Source: CAD feature listing. Evaluate the final solid. Frame: model axes, mm. A direction names the side the tool comes from. Coordinates: 2 decimals unless noted, no trailing zeros. Write each loop counter-clockwise with the first axis right and the second up, starting at its lowest first coordinate (ties: lowest second). Pieces come first, ordered by that corner, then holes. Notation, with made-up numbers: (13.25, 8) -> (42.25, 8) arc R29 cw to (42.25, 44) -> close; hole circle Ø8 at (78.5, 69). An arc over 180 degrees is marked (long way). Write item = value, one per line.
from build123d import *

# Parameters (mm, degrees)
SKETCH1_W                = 177
SKETCH1_H                = 62
BOSS_EXTRUDE1_DEPTH      = 70
FILLET1_R                = 25
SKETCH3_W                = 19
SKETCH3_H                = 17
CUT_EXTRUDE1_DEPTH       = 70
CUT_EXTRUDE5_DEPTH       = 64
BOSS_EXTRUDE7_DEPTH      = 33
SKETCH16_W               = 5
SKETCH16_H               = 5
BOSS_EXTRUDE8_DEPTH      = 40
SKETCH11_R               = 25
CUT_EXTRUDE9_DEPTH       = 5.5
SKETCH22_R               = 28.5
BOSS_EXTRUDE20_DEPTH     = 21
BOSS_EXTRUDE21_DEPTH     = 10
BOSS_EXTRUDE22_DEPTH     = 40
SKETCH26_R               = 25
SKETCH26_W               = 19
SKETCH26_H               = 17
BOSS_EXTRUDE23_DEPTH     = 1
SKETCH27_W               = 40
SKETCH27_H               = 10
CUT_EXTRUDE12_DEPTH      = 10
SKETCH28_W               = 10
SKETCH28_H               = 10
CUT_EXTRUDE13_DEPTH      = 5
SKETCH30_W               = 194.337314874
SKETCH30_H               = 68.122542634
CUT_EXTRUDE14_DEPTH      = 0.1
CUT_EXTRUDE17_DEPTH      = 58
CUT_EXTRUDE17_DEPTH_BACK = 45
SKETCH26_3_R             = 25
SKETCH26_3_W             = 19
SKETCH26_3_H             = 17
CUT_EXTRUDE25_START      = -21.9
CUT_EXTRUDE25_DEPTH      = 21.9
SKETCH38_W               = 8
SKETCH38_H               = 8
BOSS_EXTRUDE26_DEPTH     = 12
SKETCH41_R               = 3.6
CUT_EXTRUDE28_DEPTH      = 5
SKETCH44_R               = 2.1
CUT_EXTRUDE29_DEPTH      = 8
CUT_EXTRUDE30_START      = -3
SKETCH22_2_R             = 28.5
CUT_EXTRUDE30_DEPTH      = 40
SKETCH45_W               = 19.955287375
SKETCH45_H               = 24.166036088
CUT_EXTRUDE31_DEPTH      = 112


with BuildPart() as part:
    # Sketch1 → Boss-Extrude1 (new body)
    with BuildSketch(Plane(origin=(0, 0, 0), x_dir=(1, 0, 0), z_dir=(0, 1, 0))):
        with Locations((88.5, 31)):
            Rectangle(SKETCH1_W, SKETCH1_H)
    extrude(amount=BOSS_EXTRUDE1_DEPTH)

    # Fillet1
    fillet1_edges = [part.edges().sort_by_distance(p)[0] for p in [
        (0, 35, -62),
        (177, 35, -62),
        (177, 35, 0),
        (0, 35, 0),
    ]]
    fillet(fillet1_edges, radius=FILLET1_R)

    # Sketch3 → Cut-Extrude1 (cut)
    with BuildSketch(Plane(origin=(0, 70, 0), x_dir=(1, 0, 0), z_dir=(0, 1, 0))):
        with Locations((147.5, 39.5)):
            Rectangle(SKETCH3_W, SKETCH3_H)
    extrude(amount=-CUT_EXTRUDE1_DEPTH, mode=Mode.SUBTRACT)

    # Sketch9 → Cut-Extrude5 (cut)
    with BuildSketch(Plane(origin=(0, 67, 0), x_dir=(1, 0, 0), z_dir=(0, 1, 0))):
        with BuildLine():
            Line((25, 59), (152, 59))
            ThreePointArc((152, 59), (167.556349186, 52.556349186), (174, 37))
            Line((174, 37), (174, 25))
            ThreePointArc((174, 25), (167.556349186, 9.443650814), (152, 3))
            Line((152, 3), (25, 3))
            ThreePointArc((25, 3), (9.443650814, 9.443650814), (3, 25))
            Line((3, 25), (3, 37))
            ThreePointArc((3, 37), (9.443650814, 52.556349186), (25, 59))
        make_face()
    extrude(amount=-CUT_EXTRUDE5_DEPTH, mode=Mode.SUBTRACT)

    # Sketch15 → Boss-Extrude7 (add)
    with BuildSketch(Plane.XZ):
        Polygon((125, -7), (121, -3), (119, -3), (119, -7.5), (125, -7.5), align=None)
        Polygon((137, -7), (137, -7.5), (143, -7.5), (143, -3), (141, -3), align=None)
    extrude(amount=-BOSS_EXTRUDE7_DEPTH)

    # Sketch16 → Boss-Extrude8 (add)
    with BuildSketch(Plane.XZ):
        with Locations((58.5, -5.5)):
            Rectangle(SKETCH16_W, SKETCH16_H)
        Polygon((61, -40.5), (61, -44), (101, -44), (101, -40.5), (106, -40.5), (106, -59), (56, -59), (56, -40.5), align=None)
        with Locations((104.5, -5.5)):
            Rectangle(SKETCH16_W, SKETCH16_H)
    extrude(amount=-BOSS_EXTRUDE8_DEPTH)

    # Sketch11 → Cut-Extrude9 (cut)
    with BuildSketch(Plane.XZ):
        with Locations(Location((31, -31, 0), (0, 0, 270))):
            Circle(SKETCH11_R)
    extrude(amount=-CUT_EXTRUDE9_DEPTH, mode=Mode.SUBTRACT)

    # Sketch22 → Boss-Extrude20 (add)
    with BuildSketch(Plane(origin=(0, 70, 0), x_dir=(1, 0, 0), z_dir=(0, 1, 0))):
        with Locations((31, 31)):
            Circle(SKETCH22_R)
    extrude(amount=-BOSS_EXTRUDE20_DEPTH)

    # Sketch24 → Boss-Extrude21 (add)
    with BuildSketch(Plane.XZ):
        Polygon((123.5, -7.5), (125, -7.5), (125, -29.5), (137, -29.5), (137, -7.5), (138.5, -7.5), (138.5, -35.5), (123.5, -35.5), align=None)
    extrude(amount=-BOSS_EXTRUDE21_DEPTH)

    # Sketch25 → Boss-Extrude22 (add)
    with BuildSketch(Plane.XZ):
        Polygon((134.5, -35.5), (134.5, -31.5), (124.5, -31.5), (124.5, -45.5), (128.5, -45.5), (128.5, -35.5), align=None)
        Polygon((160.5, -35.5), (166.5, -35.5), (166.5, -45.5), (170.5, -45.5), (170.5, -31.5), (160.5, -31.5), align=None)
    extrude(amount=-BOSS_EXTRUDE22_DEPTH)

    # Sketch26 → Boss-Extrude23 (add)
    with BuildSketch(Plane.XZ):
        with BuildLine():
            Line((25, 0), (152, 0))
            ThreePointArc((152, 0), (169.67766953, -7.32233047), (177, -25))
            Line((177, -25), (177, -37))
            ThreePointArc((177, -37), (169.67766953, -54.67766953), (152, -62))
            Line((152, -62), (25, -62))
            ThreePointArc((25, -62), (7.32233047, -54.67766953), (0, -37))
            Line((0, -37), (0, -25))
            ThreePointArc((0, -25), (7.32233047, -7.32233047), (25, 0))
        make_face()
        with Locations(Location((31, -31, 0), (0, 0, 270))):
            Circle(SKETCH26_R, mode=Mode.SUBTRACT)
        with Locations((147.5, -39.5)):
            Rectangle(SKETCH26_W, SKETCH26_H, mode=Mode.SUBTRACT)
    extrude(amount=BOSS_EXTRUDE23_DEPTH)

    # Sketch27 → Cut-Extrude12 (cut)
    with BuildSketch(Plane.ZY):
        with Locations((-31, 34.5)):
            Rectangle(SKETCH27_W, SKETCH27_H)
    extrude(amount=-CUT_EXTRUDE12_DEPTH, mode=Mode.SUBTRACT)

    # Sketch28 → Cut-Extrude13 (cut)
    with BuildSketch(Plane.XZ.offset(1)):
        with Locations((115, -54)):
            Rectangle(SKETCH28_W, SKETCH28_H)
    extrude(amount=-CUT_EXTRUDE13_DEPTH, mode=Mode.SUBTRACT)

    # Sketch30 → Cut-Extrude14 (cut)
    with BuildSketch(Plane(origin=(0, 67, 0), x_dir=(1, 0, 0), z_dir=(0, 1, 0))):
        with Locations((88.376869027, 31.076383763)):
            Rectangle(SKETCH30_W, SKETCH30_H)
        with BuildLine():
            Line((25, 58), (152, 58))
            ThreePointArc((152, 58), (166.849242405, 51.849242405), (173, 37))
            Line((173, 37), (173, 25))
            ThreePointArc((173, 25), (166.849242405, 10.150757595), (152, 4))
            Line((152, 4), (25, 4))
            ThreePointArc((25, 4), (10.150757595, 10.150757595), (4, 25))
            Line((4, 25), (4, 37))
            ThreePointArc((4, 37), (10.150757595, 51.849242405), (25, 58))
        make_face(mode=Mode.SUBTRACT)
    extrude(amount=-CUT_EXTRUDE14_DEPTH, mode=Mode.SUBTRACT)

    # Sketch26<3> → Cut-Extrude17 (cut, two sides: drawn at the far end of the back side and taken through both)
    with BuildSketch(Plane.XZ.offset(-CUT_EXTRUDE17_DEPTH_BACK)):
        with BuildLine():
            Line((25, 0), (152, 0))
            ThreePointArc((152, 0), (169.67766953, -7.32233047), (177, -25))
            Line((177, -25), (177, -37))
            ThreePointArc((177, -37), (169.67766953, -54.67766953), (152, -62))
            Line((152, -62), (25, -62))
            ThreePointArc((25, -62), (7.32233047, -54.67766953), (0, -37))
            Line((0, -37), (0, -25))
            ThreePointArc((0, -25), (7.32233047, -7.32233047), (25, 0))
        make_face()
        with Locations((31, -31)):
            Circle(SKETCH26_3_R, mode=Mode.SUBTRACT)
        with Locations((147.5, -39.5)):
            Rectangle(SKETCH26_3_W, SKETCH26_3_H, mode=Mode.SUBTRACT)
    extrude(amount=CUT_EXTRUDE17_DEPTH + CUT_EXTRUDE17_DEPTH_BACK, mode=Mode.SUBTRACT)


with BuildPart() as cut_extrude17_piece_1:
    # of the separate pieces the step leaves, piece 1, a body of its own (cut_extrude17_pieces)
    add(part.part.solids().sort_by_distance((25, 70, 0))[0])

    # Sketch36 → Cut-Extrude25 (cut)
    with BuildSketch(Plane.XZ.offset(-45).offset(CUT_EXTRUDE25_START)):
        with BuildLine():
            Line((152, 0), (25, 0))
            ThreePointArc((25, 0), (7.32233047, -7.32233047), (0, -25))
            Line((0, -25), (0, -37))
            ThreePointArc((0, -37), (7.32233047, -54.67766953), (25, -62))
            Line((25, -62), (152, -62))
            ThreePointArc((152, -62), (169.67766953, -54.67766953), (177, -37))
            Line((177, -37), (177, -25))
            ThreePointArc((177, -25), (169.67766953, -7.32233047), (152, 0))
        make_face()
        with BuildLine():
            ThreePointArc((3, -25), (9.443650814, -9.443650814), (25, -3))
            Line((25, -3), (152, -3))
            ThreePointArc((152, -3), (167.556349186, -9.443650814), (174, -25))
            Line((174, -25), (174, -37))
            ThreePointArc((174, -37), (167.556349186, -52.556349186), (152, -59))
            Line((152, -59), (25.684927094, -59))
            ThreePointArc((25.684927094, -59), (9.884563828, -52.596687732), (3, -37))
            Line((3, -37), (3, -25))
        make_face(mode=Mode.SUBTRACT)
    extrude(amount=CUT_EXTRUDE25_DEPTH, mode=Mode.SUBTRACT)

    # Sketch38 → Boss-Extrude26 (add)
    with BuildSketch(Plane(origin=(0, 70, 0), x_dir=(1, 0, 0), z_dir=(0, 1, 0))):
        with Locations((52, 56.5)):
            Rectangle(SKETCH38_W, SKETCH38_H)
        with Locations((124, 56.5)):
            Rectangle(SKETCH38_W, SKETCH38_H)
        with Locations((52, 5.5)):
            Rectangle(SKETCH38_W, SKETCH38_H)
        with Locations((124, 5.5)):
            Rectangle(SKETCH38_W, SKETCH38_H)
    extrude(amount=-BOSS_EXTRUDE26_DEPTH)

    # Sketch41 → Cut-Extrude28 (cut)
    with BuildSketch(Plane(origin=(0, 70, 0), x_dir=(1, 0, 0), z_dir=(0, 1, 0))):
        with Locations(Location((52, 56.5, 0), (0, 0, 270))):
            Circle(SKETCH41_R)
        with Locations(Location((124, 56.5, 0), (0, 0, 270))):
            Circle(SKETCH41_R)
        with Locations(Location((52, 5.5, 0), (0, 0, 270))):
            Circle(SKETCH41_R)
        with Locations(Location((124, 5.5, 0), (0, 0, 270))):
            Circle(SKETCH41_R)
    extrude(amount=-CUT_EXTRUDE28_DEPTH, mode=Mode.SUBTRACT)

    # Sketch44 → Cut-Extrude29 (cut)
    with BuildSketch(Plane.XZ.offset(-58)):
        with Locations(Location((52, -5.5, 0), (0, 0, 270))):
            Circle(SKETCH44_R)
        with Locations(Location((124, -56.5, 0), (0, 0, 270))):
            Circle(SKETCH44_R)
        with Locations(Location((52, -56.5, 0), (0, 0, 270))):
            Circle(SKETCH44_R)
        with Locations(Location((124, -5.5, 0), (0, 0, 270))):
            Circle(SKETCH44_R)
    extrude(amount=-CUT_EXTRUDE29_DEPTH, mode=Mode.SUBTRACT)

    # Sketch22<2> → Cut-Extrude30 (cut)
    with BuildSketch(Plane(origin=(0, 70, 0), x_dir=(1, 0, 0), z_dir=(0, 1, 0)).offset(CUT_EXTRUDE30_START)):
        with Locations((31, 31)):
            Circle(SKETCH22_2_R)
    extrude(amount=-CUT_EXTRUDE30_DEPTH, mode=Mode.SUBTRACT)


with BuildPart() as cut_extrude17_piece_2:
    # of the separate pieces the step leaves, piece 2, a body of its own (cut_extrude17_pieces)
    add(part.part.solids().sort_by_distance((138.5, 0, -35.5))[0])

    # Sketch45 → Cut-Extrude31 (cut)
    with BuildSketch(Plane.XZ.offset(-67)):
        with Locations((142.415891121, -34.661520619)):
            Rectangle(SKETCH45_W, SKETCH45_H)
    extrude(amount=CUT_EXTRUDE31_DEPTH, mode=Mode.SUBTRACT)


solid = cut_extrude17_piece_1.part
1) Cut plane B-B, the plane x = 124. Output: boundary loops of the cut face in (y, z).
Answer block:
outline = (58, -60.5) -> (67, -60.5) -> (67, -62) -> (70, -62) -> (70, -60.1) -> (65, -60.1) -> (65, -58.6) -> (58, -58.6) -> close; (58, -54.4) -> (65, -54.4) -> (65, -52.9) -> (70, -52.9) -> (70, -9.1) -> (65, -9.1) -> (65, -7.6) -> (58, -7.6) -> (58, -9.5) -> (67, -9.5) -> (67, -52.5) -> (58, -52.5) -> close; (58, -3.4) -> (65, -3.4) -> (65, -1.9) -> (70, -1.9) -> (70, 0) -> (67, 0) -> (67, -1.5) -> (58, -1.5) -> close
2) Pull-direction query (Z, two-part tool) for faces 1 (the flat face through (124, 63, -52.5)), 2 (the cylindrical face through (169.871, 68.521, -54.482)), 3 (the flat face through (48, 63, -5)); classes: +Z half, -Z half, draft (parallel to the pull), parting line (faces both ways), or undercut.
Answer block:
face_1 = undercut
face_2 = -Z half
face_3 = draft
3) Cut plane C-C, the plane z = -5.5. Output: boundary loops of the cut face in (x, y).
Answer block:
outline = (9.36, 67) -> (48, 67) -> (48, 58) -> (49.9, 58) -> (49.9, 65) -> (48.4, 65) -> (48.4, 70) -> (9.36, 70) -> close; (54.1, 58) -> (56, 58) -> (56, 67) -> (120, 67) -> (120, 58) -> (121.9, 58) -> (121.9, 65) -> (120.4, 65) -> (120.4, 70) -> (55.6, 70) -> (55.6, 65) -> (54.1, 65) -> close; (126.1, 58) -> (128, 58) -> (128, 67) -> (167.64, 67) -> (167.64, 70) -> (127.6, 70) -> (127.6, 65) -> (126.1, 65) -> close
4) First-contact query: pin 1 Ø2 at (y, z) = (64, -57) entering from -X; pin 2 Ø5 at (x, z) = (52, -56.5) entering from +Y; pin 3 Ø6.5 at (x, y) = (53.5, 62.5) entering from +Z; pin 4 Ø8 at (x, z) = (125, -57.5) entering from +Y. Flat tips, straight axial feed; report the tip coordinate or a pass-through.
Answer block:
pin_1 = 48
pin_2 = 65
pin_3 = -1.5
pin_4 = 70
5) Material intervals for probe 1 along X at (y, z) = (66.15, -5.5); probe 2 along X at (y, z) = (63, -56.5); probe 3 along X at (y, z) = (67.5, -59), sorted ascending. Write a range as [from, to].
Answer block:
probe_1 = [48, 48.4], [55.6, 56], [120, 120.4], [127.6, 128]
probe_2 = [48, 49.9], [54.1, 56], [120, 121.9], [126.1, 128]
probe_3 = [13.13, 49.41], [54.59, 121.41], [126.59, 163.87]
6) Cut plane A-A, the plane y = 60.5. Output: boundary loops of the cut face in (x, z).
Answer block:
outline = (48, -60.5) -> (56, -60.5) -> (56, -52.5) -> (49.71, -52.5) arc R28.5 cw to (48, -53.87) -> close; (48, -8.13) arc R28.5 cw to (49.71, -9.5) -> (56, -9.5) -> (56, -1.5) -> (48, -1.5) -> close; (120, -60.5) -> (128, -60.5) -> (128, -52.5) -> (120, -52.5) -> close; (120, -9.5) -> (128, -9.5) -> (128, -1.5) -> (120, -1.5) -> close; hole circle Ø4.2 at (52, -56.5); hole circle Ø4.2 at (52, -5.5); hole circle Ø4.2 at (124, -56.5); hole circle Ø4.2 at (124, -5.5)
7) Cut plane D-D, the plane z = -39. Output: boundary loops of the cut face in (x, y).
Answer block:
outline = (0.08, 67) -> (138, 67) -> (138, 70) -> (0.08, 70) -> close; (157, 67) -> (176.92, 67) -> (176.92, 70) -> (157, 70) -> close
8) Reachability of faces 4 (the flat face through (120, 63, -5)), 5 (the cylindrical face through (127.57, 67.54, -5.97)), 6 (the flat face through (124, 63, -60.5)) from +Z, -Z, +X, -X, +Y, -Y: full face, straight path, thin tool, end or side. Return the list, or none.
Answer block:
face_4 = +Z, -Z, -Y
face_5 = +Y
face_6 = -Z, +X, -X, -Y
